For this review, take the finished solid that the model builds, in its own axes (mm). Coordinates: 2 decimals unless noted, no trailing zeros. Write each loop counter-clockwise with the first axis right and the second up, starting at its lowest first coordinate (ties: lowest second). Pieces come first, ordered by that corner, then holes.
1) Insertion check: P1, Ø3, axis at x = 50, z = 50, coming from the +Y side. The pin has a flat end and moves straight along its axis. Give the tip position at first contact, or say it passes through.
2) We need section B-B on x = -37.5. Write out the cut boundary in (y, z) (3 decimals), then the cut area to 3 significant figures.
3) We need section A-A on z = 0. Write out the cut boundary in (x, y) (3 decimals).
4) We need section C-C on y = 5. Give the number of separate pieces and of enclosed holes in the cut face, then the cut area to 3 significant figures.
5) To check wall thickness, follow line 1 along Z through (x, y) = (37.5, 4.25) (3 decimals); line 2 along Z through (x, y) = (50, 2) (3 decimals); line 3 along Z through (x, y) = (0, 4) (1 decimal). State the ranges of each line that lie inside material, in increasing order.
Autodesk Inventor part; units mm, degrees
ref_plane "YZ Plane" through (0, 0, 0) normal (1, 0, 0) x (0, 1, 0)
ref_plane "XZ Plane" through (0, 0, 0) normal (0, 1, 0) x (-1, 0, 0)
ref_plane "XY Plane" through (0, 0, 0) normal (0, 0, 1) x (1, 0, 0)
sketch "Sketch1" plane through (0, 0, 0) normal (0, 1, 0) x (-1, 0, 0)
  line L0 (60.325, 73.025) -> (-60.325, 73.025)
  line L1 (-73.025, 60.325) -> (-73.025, -60.325)
  line L2 (-60.325, -73.025) -> (60.325, -73.025)
  line L3 (73.025, -60.325) -> (73.025, 60.325)
  circle A0 centre (49.9999, 49.9999) radius 2
  circle A1 centre (49.9999, -49.9999) radius 2
  circle A2 centre (-49.9999, -49.9999) radius 2
  circle A3 centre (-49.9999, 49.9999) radius 2
  arc A4 (73.025, 60.325) -> (60.325, 73.025) centre (60.325, 60.325) ccw
  arc A5 (60.325, -73.025) -> (73.025, -60.325) centre (60.325, -60.325) ccw
  arc A6 (-60.325, 73.025) -> (-73.025, 60.325) centre (-60.325, 60.325) ccw
  arc A7 (-73.025, -60.325) -> (-60.325, -73.025) centre (-60.325, -60.325) ccw
  point P0 (0, 0)
  point P1 (73.025, 73.025)
  point P2 (-73.025, -73.025)
  point P3 (-73.025, 73.025)
  point P4 (73.025, -73.025)
  dimension "d0" = 73.025
  dimension "d1" = 73.025
  dimension "d2" = 146.05
  dimension "d3" = 146.05
  dimension "d4" = 4
  dimension "d5" = 4
  dimension "d6" = 4
  dimension "d7" = 4
  dimension "d8" = 99.9998
  dimension "d9" = 99.9998
  dimension "d10" = 99.9998
  dimension "d11" = 99.9998
  dimension "d12" = 23.0251
  dimension "d13" = 23.0251
  dimension "d14" = 23.0251
  dimension "d15" = 23.0251
  dimension "d16" = 23.0251
  dimension "d17" = 23.0251
  dimension "d18" = 23.0251
  dimension "d19" = 23.0251
  dimension "d40" = 12.7
  dimension "d41" = 12.7
extrude "Extrusion1" add sketch "Sketch1" along normal blind 6.35
sketch "Sketch2" plane through (0, 6.35, 0) normal (0, 1, 0) x (1, 0, 0)
  circle A0 centre (-37.5, -37.5) radius 2
  circle A1 centre (-37.5, 37.5) radius 2
  circle A2 centre (37.5, -37.5) radius 2
  circle A3 centre (37.5, 37.5) radius 2
  line L0 (-60.325, -73.025) -> (60.325, -73.025)
  line L1 (-73.025, 60.325) -> (-73.025, -60.325)
  line L2 (73.025, -60.325) -> (73.025, 60.325)
  line L3 (60.325, 73.025) -> (-60.325, 73.025)
  point P0 (0, 0)
  point P1 (-76.2, -76.2)
  point P2 (76.2, -76.2)
  point P3 (-76.2, 76.2)
  point P4 (76.2, 76.2)
  point P5 (-60.325, 73.025)
  dimension "d22" = 4
  dimension "d23" = 4
  dimension "d24" = 4
  dimension "d25" = 4
  dimension "d26" = 75
  dimension "d27" = 75
  dimension "d28" = 75
  dimension "d29" = 75
  dimension "d30" = 35.525
  dimension "d31" = 35.525
  dimension "d32" = 35.525
  dimension "d33" = 35.525
  dimension "d34" = 35.525
  dimension "d35" = 35.525
  dimension "d36" = 35.525
  dimension "d37" = 35.525
extrude "Extrusion2" cut sketch "Sketch2" against normal blind 6.35
sketch "Sketch3" plane through (0, 6.35, 0) normal (0, 1, 0) x (1, 0, 0)
  circle A0 centre (0, -36.5125) radius 3.302
  circle A1 centre (0, 0) radius 3.302
  circle A2 centre (0, 36.5125) radius 3.302
  line L0 (60.325, 73.025) -> (-60.325, 73.025)
  line L1 (-60.325, -73.025) -> (60.325, -73.025)
  line L2 (73.025, -60.325) -> (73.025, 60.325)
  line L3 (-73.025, 60.325) -> (-73.025, -60.325)
  point P0 (-73.025, 0)
  dimension "d52" = 6.604
  dimension "d53" = 6.604
  dimension "d54" = 6.604
  dimension "d61" = 36.5125
  dimension "d62" = 36.5125
  dimension "d63" = 36.5125
  dimension "d64" = 36.5125
extrude "Extrusion3" cut sketch "Sketch3" against normal blind 6.35
ref_plane "Work Plane1" through (0, 0, 60.325) normal (1, 0, 0) x (0, 0, -1)
ref_plane "Work Plane2" through (-60.325, 0, 0) normal (0, 0, 1) x (1, 0, 0)
equation "\"d5\" = d4"
equation "\"d6\" = d4"
equation "\"d7\" = d4"
equation "\"d9\" = d8"
equation "\"d11\" = d10"
equation "\"d12\" = d17"
equation "\"d13\" = d16"
equation "\"d14\" = d13"
equation "\"d15\" = d12"
equation "\"d23\" = d22"
equation "\"d24\" = d22"
equation "\"d25\" = d22"
equation "\"d27\" = d26"
equation "\"d29\" = d28"
equation "\"d30\" = d36"
equation "\"d31\" = d37"
equation "\"d32\" = d31"
equation "\"d33\" = d30"
equation "\"d52\" = d53"
equation "\"d54\" = d53"
properties part number "VESA adapter bracket"
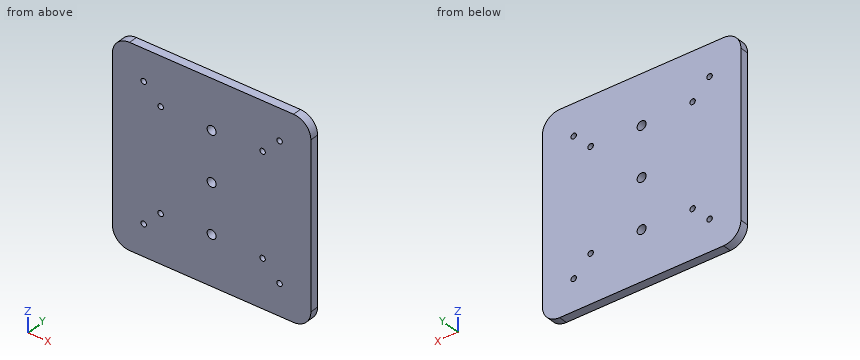
Result:
1. P1: passes through
2. outline: (0, -73.025) - (6.35, -73.025) - (6.35, -39.5) - (0, -39.5) - close; (0, -35.5) - (6.35, -35.5) - (6.35, 35.5) - (0, 35.5) - close; (0, 39.5) - (6.35, 39.5) - (6.35, 73.025) - (0, 73.025) - close
2. area: 877 mm2
3. outline: (-73.025, 0) - (-3.302, 0) - (-3.302, 6.35) - (-73.025, 6.35) - close; (3.302, 0) - (73.025, 0) - (73.025, 6.35) - (3.302, 6.35) - close
4. separate pieces: 1
4. enclosed holes: 11
4. area: 21,000 mm2
5. line 1: z = -73.025 to -39.5, -35.5 to 35.5, 39.5 to 73.025
5. line 2: z = -73.025 to -52, -48 to 48, 52 to 73.025
5. line 3: z = -73 to -39.8, -33.2 to -3.3, 3.3 to 33.2, 39.8 to 73
